from build123d import *

# Parameters (mm, degrees)
SKETCH1_W           = 500
SKETCH1_H           = 300
BOSS_EXTRUDE1_DEPTH = 10
SKETCH2_W           = 10
SKETCH2_H           = 60
EXTRUDE_THIN1_DEPTH = 500
SKETCH3_R           = 7.5
CUT_EXTRUDE1_DEPTH  = 403.740611312
FILLET1_R           = 10


with BuildPart() as part:
    # Sketch1 → Boss-Extrude1 (new body)
    with BuildSketch(Plane(origin=(0, 0, 0), x_dir=(0, 1, 0), z_dir=(0, 0, 1))):
        Rectangle(SKETCH1_W, SKETCH1_H)
    extrude(amount=BOSS_EXTRUDE1_DEPTH)

    # Sketch2 → Extrude-Thin1 (add)
    with BuildSketch(Plane.XZ.offset(250)):
        with Locations((-150, 30)):
            Rectangle(SKETCH2_W, SKETCH2_H)
        with Locations((150, 30)):
            Rectangle(SKETCH2_W, SKETCH2_H)
    extrude(amount=-EXTRUDE_THIN1_DEPTH)

    # Sketch3 → Cut-Extrude1 (cut, through all)
    with BuildSketch(Plane.YZ.offset(155)):
        with Locations(Location((-220, 30, 0), (0, 0, 270))):
            Circle(SKETCH3_R)
        with BuildLine():
            Line((-30, 37.5), (220, 37.5))
            ThreePointArc((220, 37.5), (227.5, 30), (220, 22.5))
            Line((220, 22.5), (-30, 22.5))
            ThreePointArc((-30, 22.5), (-37.5, 30), (-30, 37.5))
        make_face()
    extrude(amount=-CUT_EXTRUDE1_DEPTH, mode=Mode.SUBTRACT)

    # Fillet1
    fillet1_edges = [part.edges().sort_by_distance(p)[0] for p in [
        (-150, 250, 60),
        (-150, -250, 60),
        (150, 250, 60),
        (150, -250, 60),
    ]]
    fillet(fillet1_edges, radius=FILLET1_R)


solid = part.part
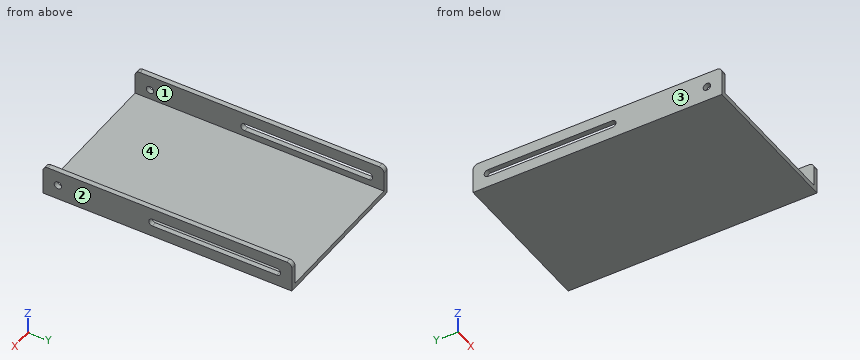
Geometry: final body of the model. Coordinates: model frame, mm. Face numbers are marked on the shaded views. Give positions to 0.01 mm unless a question says otherwise; leave off trailing zeros. Write each loop counter-clockwise with the first axis right and the second up, starting at its lowest first coordinate (ties: lowest second). Pieces come first, ordered by that corner, then holes. Notation, with made-up numbers: (15, 88.25) -> (19, 88.25) arc R9 ccw to (19, 105.25) -> close; hole circle Ø1 at (58, 72). An arc over 180 degrees is marked (long way). Answer as a JSON object with one key per item and string values.
1. Ray query, probe 1 along Y at (x, z) = (-150.75, 30); probe 2 along X at (y, z) = (130.5, 40); probe 3 along Z at (x, y) = (81.5, 197.5). Return the intervals inside material, ascending. Write a range as from..to.
Ans:
{"probe 1": "y = -250..-227.5, -212.5..-37.5, 227.5..250", "probe 2": "x = -155..-145, 145..155", "probe 3": "z = 0..10"}
2. Contact query for a flat-ended pin moving along its axis: pin 1 (6 mm diameter, centred on x = 20.5, y = 195.5, fed in from +Z). Output: stop coordinate, or through.
Ans:
{"pin 1": "stops at z = 10"}
3. Cut plane B-B on z = 30. Output: boundary loops of the cut face in (x, y), and give its area (3 significant figures).
Ans:
{"outline": "(-155, -250) -> (-145, -250) -> (-145, -227.5) -> (-155, -227.5) -> close; (-155, -212.5) -> (-145, -212.5) -> (-145, -37.5) -> (-155, -37.5) -> close; (-155, 227.5) -> (-145, 227.5) -> (-145, 250) -> (-155, 250) -> close; (145, -250) -> (155, -250) -> (155, -227.5) -> (145, -227.5) -> close; (145, -212.5) -> (155, -212.5) -> (155, -37.5) -> (145, -37.5) -> close; (145, 227.5) -> (155, 227.5) -> (155, 250) -> (145, 250) -> close", "area": "4,400 mm^2"}
4. Cut plane D-D on x = -105. Output: boundary loops of the cut face in (y, z), and give its area (3 significant figures).
Ans:
{"outline": "(-250, 0) -> (250, 0) -> (250, 10) -> (-250, 10) -> close", "area": "5,000 mm^2"}
5. Cut plane C-C on y = -181. Output: boundary loops of the cut face in (x, z).
Ans:
{"outline": "(-155, 0) -> (155, 0) -> (155, 60) -> (145, 60) -> (145, 10) -> (-145, 10) -> (-145, 60) -> (-155, 60) -> close"}
6. Mould query, pull axis X, two halves, no side actions, for the marked faces 1, 2, 3 and 4. Classes: pulls with the +X half, pulls with the -X half, needs draft (parallel to the pull), parting line crosses it, or undercut.
Ans:
{"face 1": "undercut", "face 2": "pulls with the +X half", "face 3": "pulls with the -X half", "face 4": "undercut"}
7. Cut plane A-A on y = 134. Output: boundary loops of the cut face in (x, z).
Ans:
{"outline": "(-155, 0) -> (155, 0) -> (155, 22.5) -> (145, 22.5) -> (145, 10) -> (-145, 10) -> (-145, 22.5) -> (-155, 22.5) -> close; (-155, 37.5) -> (-145, 37.5) -> (-145, 60) -> (-155, 60) -> close; (145, 37.5) -> (155, 37.5) -> (155, 60) -> (145, 60) -> close"}
